Could you check a few things on this model? Use its own coordinates, in mm. A direction names the side the tool comes from. Round coordinates to 2 decimals unless told otherwise and drop trailing zeros. Write each loop counter-clockwise with the first axis right and the second up, starting at its lowest first coordinate (ties: lowest second). Pieces come first, ordered by that corner, then holes. Notation, with made-up numbers: (27, -16) -> (81, -16) arc R22 cw to (81, 15) -> close; hole circle Ø11 at (7, 62). An arc over 180 degrees is marked (long way). Answer as CSV lines item,"result". Start each with the question number.
Q1. Imagine slicing it at C-C on y = 8.5. Please give me the cut outline in (x, z).
Q2. If we mould it in two halves opening along X, with no side actions, what happens to faces 1 (the cylindrical face through (-10.74, 13.74, -2.38)), 2 (the flat face through (-7.3, 2, -5.8)), 3 (the cylindrical face through (-2.44, 11.34, -0.54))? For each: pulls with the +X half, pulls with the -X half, needs draft (parallel to the pull), parting line crosses it, or undercut.
Q3. Will these pins go through, and if not, where does the flat tip stop? pin 1 Ø1.5 at (y, z) = (9.5, -5.5) entering from +X; pin 2 Ø1 at (x, z) = (3, -4.5) entering from -Y; pin 3 Ø5 at (x, y) = (-2, 19) entering from -Z; pin 4 Ø4 at (x, y) = (-5, 8.5) entering from +Z.
Q4. Imagine slicing it at B-B on x = 0. Please give me the cut outline in (y, z), and give its area (3 significant figures).
Q5. If I drill on line 1 (Y direction, x = 5.5, z = -7.75); line 2 (X direction, y = 14.25, z = 0); line 3 (X direction, y = 9.5, z = 0), over which ranges is the centre line in solid material (lowest first)? Write a range as [from, to].
Q6. Imagine slicing it at A-A on z = 0. Please give me the cut outline in (x, y), and give its area (3 significant figures).
Q7. For faces 4 (the cylindrical face through (2.75, 7.42, 8.75)), 5 (the flat face through (-2, 0, 2)), 6 (the flat face through (-7, 15, 5)), which set-ups out of +Z, -Z, +X, -X, +Y, -Y let a thin tool reach every point of the face, with its end or its side?
from build123d import *

# Parameters (mm, degrees)
SKETCH_1_R          = 11
SKETCH_1_R_2        = 2.5
EXTRUDE_1_DEPTH     = 15
SKETCH_2_R          = 7.5
SKETCH_2_R_2        = 2.5
EXTRUDE_2_DEPTH     = 8
CUT_EXTRUDE_START   = 2
SKETCH_3_R          = 11
SKETCH_3_R_2        = 9.17
CUT_EXTRUDE_1_DEPTH = 11
FILLET_1_R          = 0.5


with BuildPart() as part:
    # 草图1 → 凸台-拉伸1 (new body)
    with BuildSketch(Plane(origin=(0, 0, 0), x_dir=(1, 0, 0), z_dir=(0, 1, 0))):
        with Locations(Location((0, 0, 0), (0, 0, 270))):
            Circle(SKETCH_1_R)
        with Locations(Location((0, 0, 0), (0, 0, 270))):
            Circle(SKETCH_1_R_2, mode=Mode.SUBTRACT)
    extrude(amount=EXTRUDE_1_DEPTH)

    # 草图2 → 凸台-拉伸2 (add)
    with BuildSketch(Plane(origin=(0, 15, 0), x_dir=(1, 0, 0), z_dir=(0, 1, 0))):
        with Locations(Location((0, 0, 0), (0, 0, 270))):
            Circle(SKETCH_2_R)
        with Locations(Location((0, 0, 0), (0, 0, 270))):
            Circle(SKETCH_2_R_2, mode=Mode.SUBTRACT)
    extrude(amount=EXTRUDE_2_DEPTH)

    # 草图3 → 切除-拉伸1 (cut)
    with BuildSketch(Plane(origin=(0, 0, 0), x_dir=(1, 0, 0), z_dir=(0, 1, 0)).offset(CUT_EXTRUDE_START)):
        with Locations(Location((0, 0, 0), (0, 0, 270))):
            Circle(SKETCH_3_R)
        with Locations(Location((0, 0, 0), (0, 0, 270))):
            Circle(SKETCH_3_R_2, mode=Mode.SUBTRACT)
    extrude(amount=CUT_EXTRUDE_1_DEPTH, mode=Mode.SUBTRACT)

    # 圆角1
    fillet_1_edges = [part.edges().sort_by_distance(p)[0] for p in [
        (0, 0, -11),
        (0, 15, -11),
        (0, 23, -7.5),
    ]]
    fillet(fillet_1_edges, radius=FILLET_1_R)


solid = part.part
Checks:
1,outline,"circle Ø18.34 at (0, 0); hole circle Ø5 at (0, 0)"
2,face 1,"parting line crosses it"
2,face 2,"needs draft"
2,face 3,"undercut"
3,pin 1,"x = 7.84"
3,pin 2,"y = 0"
3,pin 3,"z = -7.5"
3,pin 4,"z = 8.67"
4,outline,"(0, -10.5) arc R0.5 ccw to (0.5, -11) -> (2, -11) -> (2, -9.17) -> (13, -9.17) -> (13, -11) -> (14.5, -11) arc R0.5 ccw to (15, -10.5) -> (15, -7.5) -> (22.5, -7.5) arc R0.5 ccw to (23, -7) -> (23, -2.5) -> (0, -2.5) -> close; (0, 2.5) -> (23, 2.5) -> (23, 7) arc R0.5 ccw to (22.5, 7.5) -> (15, 7.5) -> (15, 10.5) arc R0.5 ccw to (14.5, 11) -> (13, 11) -> (13, 9.17) -> (2, 9.17) -> (2, 11) -> (0.5, 11) arc R0.5 ccw to (0, 10.5) -> close"
4,area,"294 mm^2"
5,line 1,"[0, 2], [13, 15]"
5,line 2,"[-11, -2.5], [2.5, 11]"
5,line 3,"[-9.17, -2.5], [2.5, 9.17]"
6,outline,"(-11, 0.5) arc R0.5 ccw to (-10.5, 0) -> (-2.5, 0) -> (-2.5, 23) -> (-7, 23) arc R0.5 ccw to (-7.5, 22.5) -> (-7.5, 15) -> (-10.5, 15) arc R0.5 ccw to (-11, 14.5) -> (-11, 13) -> (-9.17, 13) -> (-9.17, 2) -> (-11, 2) -> close; (2.5, 0) -> (10.5, 0) arc R0.5 ccw to (11, 0.5) -> (11, 2) -> (9.17, 2) -> (9.17, 13) -> (11, 13) -> (11, 14.5) arc R0.5 ccw to (10.5, 15) -> (7.5, 15) -> (7.5, 22.5) arc R0.5 ccw to (7, 23) -> (2.5, 23) -> close"
6,area,"294 mm^2"
7,face 4,"none"
7,face 5,"+Z, -Z, +X, -X, -Y"
7,face 6,"+Y"
